Source: CAD feature listing. Evaluate the final solid. Frame: model axes, mm. Give positions to 0.01 mm unless a question says otherwise; leave off trailing zeros. Order: outer loops, then holes, each group sorted by start corner. A loop starts at its lowest first (then second) coordinate and runs counter-clockwise, first axis right, second up. Notation, with made-up numbers: (1.25, -9.75) - (52.25, -9.75) arc R13 cw to (52.25, 11.25) - close; hole circle Ø6 at (66, -18.5). An arc over 180 degrees is marked (long way). One line per item, written item: value. Start each with the question number.
from build123d import *

# Parameters (mm, degrees)
BOSS_EXTRUDE1_DEPTH     = 5
SKETCH2_OUTSIDE_W       = 45.342
SKETCH2_OUTSIDE_H       = 43.33
SKETCH2_OUTSIDE_R       = 6.5
CUT_EXTRUDE1_DEPTH      = 12.116804097
CUT_EXTRUDE1_DRAFT      = -45
MIRROR1_COPY_1_SKETCH_W = 45.342
MIRROR1_COPY_1_SKETCH_H = 43.33
MIRROR1_COPY_1_SKETCH_R = 6.5
MIRROR1_COPY_1_DEPTH    = 12.116804097
MIRROR1_COPY_1_DRAFT    = -45
SKETCH3_R               = 4
CUT_EXTRUDE2_DEPTH      = 12.116804097


with BuildPart() as part:
    # Sketch1 → Boss-Extrude1 (new body)
    with BuildSketch(Plane(origin=(0, 0, 0), x_dir=(1, 0, 0), z_dir=(0, 1, 0))):
        Polygon((7.505553499, 0), (3.75277675, 6.5), (-3.75277675, 6.5), (-7.505553499, 0), (-3.75277675, -6.5), (3.75277675, -6.5), align=None)
    extrude(amount=BOSS_EXTRUDE1_DEPTH)


with BuildPart() as cut_extrude1_tool:
    # Sketch2 outside → Cut-Extrude1 (with draft: the straight prism first)
    with BuildSketch(Plane(origin=(0, 5, 0), x_dir=(1, 0, 0), z_dir=(0, 1, 0))):
        Rectangle(SKETCH2_OUTSIDE_W, SKETCH2_OUTSIDE_H)
        Circle(SKETCH2_OUTSIDE_R, mode=Mode.SUBTRACT)
    extrude(amount=-CUT_EXTRUDE1_DEPTH)
    # Cut-Extrude1: the draft: its side faces are tilted about the plane it starts from
    cut_extrude1_sides = [cut_extrude1_tool.faces().sort_by_distance(p)[0] for p in [
        (0, -1.058402049, 21.665),
        (22.671, -1.058402049, 0),
        (0, -1.058402049, -21.665),
        (-22.671, -1.058402049, 0),
        (-6.5, -1.058402049, 0),
    ]]
    draft(cut_extrude1_sides, Plane(origin=(0, 5, 0), x_dir=(1, 0, 0), z_dir=(0, 1, 0)), CUT_EXTRUDE1_DRAFT)


with BuildPart() as part_1:
    add(part.part)

    # Cut-Extrude1: cut by cut_extrude1_tool
    add(cut_extrude1_tool.part, mode=Mode.SUBTRACT)


with BuildPart() as mirror1_copy_1_tool:
    # Mirror1 copy 1 sketch → Mirror1 copy 1 (with draft: the straight prism first)
    with BuildSketch(Plane.XZ):
        Rectangle(MIRROR1_COPY_1_SKETCH_W, MIRROR1_COPY_1_SKETCH_H)
        Circle(MIRROR1_COPY_1_SKETCH_R, mode=Mode.SUBTRACT)
    extrude(amount=-MIRROR1_COPY_1_DEPTH)
    # Mirror1 copy 1: the draft: its side faces are tilted about the plane it starts from
    mirror1_copy_1_sides = [mirror1_copy_1_tool.faces().sort_by_distance(p)[0] for p in [
        (0, 6.058402049, 21.665),
        (22.671, 6.058402049, 0),
        (0, 6.058402049, -21.665),
        (-22.671, 6.058402049, 0),
        (-6.5, 6.058402049, 0),
    ]]
    draft(mirror1_copy_1_sides, Plane.XZ, MIRROR1_COPY_1_DRAFT)


with BuildPart() as part_2:
    add(part_1.part)

    # Mirror1 copy 1: cut by mirror1_copy_1_tool
    add(mirror1_copy_1_tool.part, mode=Mode.SUBTRACT)

    # Sketch3 → Cut-Extrude2 (cut, through all)
    with BuildSketch(Plane(origin=(0, 5, 0), x_dir=(1, 0, 0), z_dir=(0, 1, 0))):
        with Locations(Location((0, 0, 0), (0, 0, 270))):
            Circle(SKETCH3_R)
    extrude(amount=-CUT_EXTRUDE2_DEPTH, mode=Mode.SUBTRACT)


solid = part_2.part
1. Draft query along Z for faces 1 (the flat face through (0, 2, 6.5)), 2 (the cylindrical face through (-3.905, 2.535, -0.867)), 3 (the conical face through (-3.36, 4.76, -5.84)), 4 (the conical face through (-6.7, 4.8, 0)). Return one class per face: pulls with the +Z half, pulls with the -Z half, needs draft (parallel to the pull), parting line crosses it, or undercut.
2. Contact query for a flat-ended pin moving along its axis: pin 1 Ø2 at (x, y) = (-5.5, 4.5) entering from -Z. Output: stop coordinate, or through.
3. Section A-A on y = 2.1. Return the cut outline in (x, z), then the cut area to 3 significant figures.
4. Ray query, L1, parallel to Z at x = 1.5, y = 2.5; L2, parallel to X at y = 1.5, z = 2.5; L3, parallel to X at y = 4.6, z = -2.25. Return the intervals inside material, ascending.
Data:
1. face 1: pulls with the +Z half
1. face 2: undercut
1. face 3: pulls with the -Z half
1. face 4: parting line crosses it
2. pin 1: stops at z = -5.21
3. outline: (-7.51, 0) - (-3.75, -6.5) - (3.75, -6.5) - (7.51, 0) - (3.75, 6.5) - (-3.75, 6.5) - close; hole circle Ø8 at (0, 0)
3. area: 96.1 mm2
4. L1: z = -6.5 to -3.71, 3.71 to 6.5
4. L2: x = -6.06 to -3.12, 3.12 to 6.06
4. L3: x = -6.21 to -3.31, 3.31 to 6.21
